```python
from build123d import *

# Parameters (mm, degrees)
BOSS_EXTRUDE1_DEPTH                  = 4.7625
BOSS_EXTRUDE1_DEPTH_BACK             = 2.38125
SKETCH1_R                            = 4.7625
SKETCH1_R_2                          = 3.175
SKETCH2_R                            = 2.38125
BOSS_EXTRUDE2_DEPTH                  = 28.575
BOSS_EXTRUDE2_DIRECTION_2_REACH      = 13.666
BOSS_EXTRUDE2_DIRECTION_2_END_RADIUS = 4.7625
SKETCH3_W                            = 3.175
SKETCH3_H                            = 1.5875
BOSS_EXTRUDE3_START                  = 25.4
SKETCH4_R                            = 2.38125
BOSS_EXTRUDE3_DEPTH                  = 25.4
SKETCH5_R                            = 3.175
BOSS_EXTRUDE4_DEPTH                  = 3.175
SKETCH6_R                            = 1.5875
BOSS_EXTRUDE5_DEPTH                  = 0.83185
SKETCH7_W                            = 15.534712676
SKETCH7_H                            = 81.822586025
CUT_EXTRUDE1_DEPTH                   = 74.056725452


with BuildPart() as part:
    # Sketch1 → Boss-Extrude1 (new, two sides: drawn at the far end of the back side and taken through both)
    with BuildSketch(Plane.XY.offset(-BOSS_EXTRUDE1_DEPTH_BACK)):
        Circle(SKETCH1_R)
        Circle(SKETCH1_R_2, mode=Mode.SUBTRACT)
    extrude(amount=BOSS_EXTRUDE1_DEPTH + BOSS_EXTRUDE1_DEPTH_BACK)

    # Sketch2 → Boss-Extrude2 (add)
    with BuildSketch(Plane(origin=(0, 4.7625, 0), x_dir=(1, 0, 0), z_dir=(0, 1, 0))):
        with Locations(Location((0, 0, 0), (0, 0, 90.000000028))):
            Circle(SKETCH2_R)
    extrude(amount=BOSS_EXTRUDE2_DEPTH)

    # Boss-Extrude2 direction 2: up to this cylinder (the profile starts outside it)
    boss_extrude2_direction_2_end = Plane(origin=(0, 0, 0), z_dir=(0, 0, 1)) * Cylinder(BOSS_EXTRUDE2_DIRECTION_2_END_RADIUS, 37.857, mode=Mode.PRIVATE)
    # Sketch2 → Boss-Extrude2 direction 2 (add, up to the surface)
    with BuildSketch(Plane(origin=(0, 4.7625, 0), x_dir=(1, 0, 0), z_dir=(0, 1, 0)), mode=Mode.PRIVATE) as boss_extrude2_direction_2_sk1:
        with Locations(Location((0, 0, 0), (0, 0, 90.000000028))):
            Circle(SKETCH2_R)
    boss_extrude2_direction_2_tool1 = extrude(boss_extrude2_direction_2_sk1.sketch, amount=-BOSS_EXTRUDE2_DIRECTION_2_REACH, mode=Mode.PRIVATE) - boss_extrude2_direction_2_end
    add(boss_extrude2_direction_2_tool1.solids().sort_by_distance((0, 4.7625, 0))[0])
    add(boss_extrude2_direction_2_tool1.solids().sort_by_distance((0, 4.7625, 0))[1])

    # Sketch3 → Revolve1 (revolve)
    with BuildSketch(Plane(origin=(0, 0, 0), x_dir=(0, 0, -1), z_dir=(1, 0, 0)), mode=Mode.PRIVATE) as revolve1_sk:
        with Locations((-1.5875, 33.3375)):
            Rectangle(SKETCH3_W, SKETCH3_H)
        Polygon((-2.921, 34.76625), (-2.921, 34.13125), (0, 34.13125), (0, 43.33875), (-3.175, 43.33875), (-3.175, 41.75125), (-2.921, 41.75125), (-2.921, 41.11625), (-3.96875, 40.3225), (-2.921, 39.52875), (-3.96875, 38.735), (-2.921, 37.94125), (-3.96875, 37.1475), (-2.921, 36.35375), (-3.96875, 35.56), align=None)
    revolve(revolve1_sk.sketch.rotate(Axis((0, 32.54375, 0), (0, 1, 0)), 180), axis=Axis((0, 32.54375, 0), (0, 1, 0)))

    # Sketch4 → Boss-Extrude3 (add)
    with BuildSketch(Plane(origin=(0, 43.33875, 0), x_dir=(1, 0, 0), z_dir=(0, 1, 0)).offset(BOSS_EXTRUDE3_START)):
        with Locations(Location((0, 0, 0), (0, 0, 90))):
            Circle(SKETCH4_R)
    extrude(amount=-BOSS_EXTRUDE3_DEPTH)

    # Sketch5 → Boss-Extrude4 (add)
    with BuildSketch(Plane(origin=(0, 68.73875, 0), x_dir=(1, 0, 0), z_dir=(0, 1, 0))):
        with Locations(Location((0, 0, 0), (0, 0, 90))):
            Circle(SKETCH5_R)
    extrude(amount=BOSS_EXTRUDE4_DEPTH)

    # Sketch6 → Boss-Extrude5 (add)
    with BuildSketch(Plane(origin=(0, 71.91375, 0), x_dir=(1, 0, 0), z_dir=(0, 1, 0))):
        with Locations(Location((0, 0, 0), (0, 0, 270))):
            Circle(SKETCH6_R)
    extrude(amount=BOSS_EXTRUDE5_DEPTH)

    # Sketch7 → Cut-Extrude1 (cut, through all)
    with BuildSketch(Plane.XY):
        with Locations((0.627177841, 34.425750044)):
            Rectangle(SKETCH7_W, SKETCH7_H)
    extrude(amount=-CUT_EXTRUDE1_DEPTH, mode=Mode.SUBTRACT)


solid = part.part
```
Verification items for the finished model (mm, model axes). A direction names the side the tool comes from. Give positions to 0.01 mm unless a question says otherwise; leave off trailing zeros. Order: outer loops, then holes, each group sorted by start corner. A loop starts at its lowest first (then second) coordinate and runs counter-clockwise, first axis right, second up. Notation, with made-up numbers: M 66.25,39.5 L 113.25,39.5 A22 ccw 113.25,75.5 Z; hole C 52.5,69 d8. An arc over 180 degrees is marked long. Answer in a Markdown table with one row per item. Add a question column.
Item 1: Scan lines: probe 1 along Y at (x, z) = (0, 2.6) (1 decimal); probe 2 along X at (y, z) = (0, 1.9) (1 decimal); probe 3 along Y at (x, z) = (0, 1.4) (1 decimal). Record each from-to range of solid material in increasing order. Write a range as from..to.
Item 2: Gauge pin test, flat ends, axial feed: pin 1 (1.5 mm diameter, centred on x = 3.5, z = 1.5, fed in from +Y); pin 2 (5 mm diameter, centred on x = 0, y = 0, fed in from +Z). Record the tip position at first contact, or that the pin passes through.
Item 3: Mould release check, pull along Y, two halves, no side actions. Record for faces 1 (the cylindrical face through (-0.07, 70.304, 3.174)), 2 (the cylindrical face through (-1.03, -4.65, 2.35)), 3 (the flat face through (0, 71.914, 2)): released by +Y, released by -Y, zero draft, split by the parting line, or undercut.
Item 4: Tool access check on faces 4 (the flat face through (0, 35, 0)), 5 (the cylindrical face through (-0.07, 33.349, 3.174)), 6 (the cylindrical face through (-0.035, 72.324, 1.587)). Record the directions out of +Z, -Z, +X, -X, +Y, -Y that give a thin tool (end or side, any length) a straight path to the whole face; none if there is none.
Item 5: Section check A-A, the plane y = 0. Enter the section's corners in (x, z) (1 decimal), and give its area (3 significant figures).
Filled sheet:
| question | item | result |
|---|---|---|
| 1 | probe 1 | y = -4.8..-3.2, 3.2..4.8, 32.5..43.3, 68.7..71.9 |
| 1 | probe 2 | x = -4.8..-3.2, 3.2..4.8 |
| 1 | probe 3 | y = -4.8..-3.2, 3.2..72.7 |
| 2 | pin 1 | stops at y = 71.91 |
| 2 | pin 2 | passes through |
| 3 | face 1 | zero draft |
| 3 | face 2 | undercut |
| 3 | face 3 | released by +Y |
| 4 | face 4 | -Z, +X, -X, +Y, -Y |
| 4 | face 5 | +Z |
| 4 | face 6 | +Z, +Y |
| 5 | outline | M -4.8,0 L -3.2,0 L -3.2,4.8 L -4.8,4.8 Z; M 3.2,0 L 4.8,0 L 4.8,4.8 L 3.2,4.8 Z |
| 5 | area | 15.1 mm^2 |
